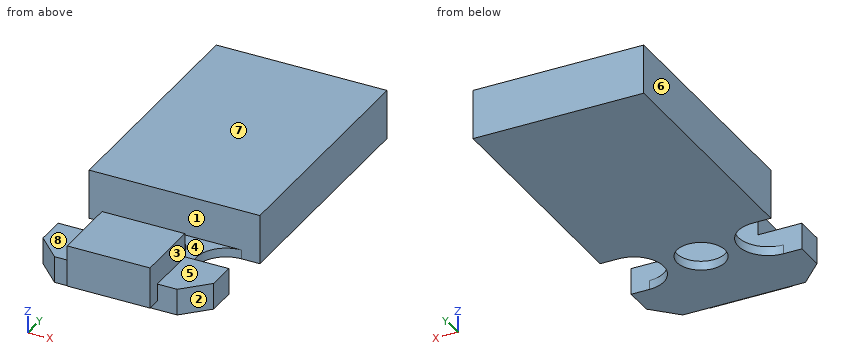
```python
from build123d import *

# Parameters (mm, degrees)
SKETCH1_W           = 20.6
SKETCH1_H           = 43.1
BOSS_EXTRUDE1_DEPTH = 1.1
SKETCH2_W           = 20.6
SKETCH2_H           = 29.5
BOSS_EXTRUDE2_DEPTH = 4.9
SKETCH3_R           = 2.9
CUT_EXTRUDE1_DEPTH  = 4.9
SKETCH4_W           = 10
SKETCH4_H           = 8.1
BOSS_EXTRUDE3_DEPTH = 5
SKETCH5_W           = 20.6
SKETCH5_H           = 6.4
BOSS_EXTRUDE4_DEPTH = 2.1
CUT_EXTRUDE2_DEPTH  = 48.877029983


with BuildPart() as part:
    # Sketch1 → Boss-Extrude1 (new body)
    with BuildSketch(Plane.XY):
        with Locations((10.3, 21.55)):
            Rectangle(SKETCH1_W, SKETCH1_H)
    extrude(amount=BOSS_EXTRUDE1_DEPTH)

    # Sketch2 → Boss-Extrude2 (add)
    with BuildSketch(Plane.XY.offset(1.1)):
        with Locations((10.3, 28.35)):
            Rectangle(SKETCH2_W, SKETCH2_H)
    extrude(amount=BOSS_EXTRUDE2_DEPTH)

    # Sketch3 → Cut-Extrude1 (cut)
    with BuildSketch(Plane.XY.offset(1.1)):
        with Locations((10.3, 10)):
            Circle(SKETCH3_R)
        with BuildLine():
            Line((0, 13.6), (2.2, 13.6))
            ThreePointArc((2.2, 13.6), (5.8, 10), (2.2, 6.4))
            Line((2.2, 6.4), (0, 6.4))
            Line((0, 6.4), (0, 13.6))
        make_face()
        with BuildLine():
            Line((20.6, 13.6), (18.4, 13.6))
            ThreePointArc((18.4, 13.6), (14.8, 10), (18.4, 6.4))
            Line((18.4, 6.4), (20.6, 6.4))
            Line((20.6, 6.4), (20.6, 13.6))
        make_face()
    extrude(amount=-CUT_EXTRUDE1_DEPTH, mode=Mode.SUBTRACT)

    # Sketch4 → Boss-Extrude3 (add)
    with BuildSketch(Plane.XY.offset(1.1)):
        with Locations((10.3, 2.35)):
            Rectangle(SKETCH4_W, SKETCH4_H)
    extrude(amount=BOSS_EXTRUDE3_DEPTH)

    # Sketch5 → Boss-Extrude4 (add)
    with BuildSketch(Plane.XY.offset(1.1)):
        with Locations((10.3, 3.2)):
            Rectangle(SKETCH5_W, SKETCH5_H)
    extrude(amount=BOSS_EXTRUDE4_DEPTH)

    # Sketch6 → Cut-Extrude2 (cut, through all)
    with BuildSketch(Plane.XY.offset(3.2)):
        Polygon((0, 0), (0, 2.9), (2.9, 0), align=None)
        Polygon((20.6, 0), (20.6, 2.9), (17.7, 0), align=None)
    extrude(amount=-CUT_EXTRUDE2_DEPTH, mode=Mode.SUBTRACT)


solid = part.part
```
Geometry check sheet. Reference: the model listing, model coordinates, mm. Face numbers are marked on the shaded views. A direction names the side the tool comes from. Give positions to 0.01 mm unless a question says otherwise; leave off trailing zeros. Write each loop counter-clockwise with the first axis right and the second up, starting at its lowest first coordinate (ties: lowest second). Pieces come first, ordered by that corner, then holes.
1) Material ranges on L1, parallel to Y at x = 10.3, z = 0.35; L2, parallel to Y at x = 14.5, z = 2.25; L3, parallel to Z at x = 8.75, y = 41.5, recorded low to high.
2) Gauge pin test, flat ends, axial feed: pin 1 (1.5 mm diameter, centred on y = 3.5, z = 4, fed in from -X); pin 2 (8 mm diameter, centred on x = 10, y = 37, fed in from +Z); pin 3 (6 mm diameter, centred on x = 2, y = 3, fed in from +Z); pin 4 (9.5 mm diameter, centred on x = 10.3, y = 10, fed in from +Z). Record the tip position at first contact, or that the pin passes through.
3) Section check D-D, the plane y = 5.5. Record the boundary of the cut face in (x, z), and give its area (3 significant figures).
4) Section check B-B, the plane y = 10. Record the boundary of the cut face in (x, z), and give its area (3 significant figures).
5) Access from +Z, -Z, +X, -X, +Y, -Y to the whole of each face (thin tool, end or side, straight path). Record for the marked faces 4, 5, 6, 7 and 8.
6) Release check for a two-part mould opening along Y. For the marked faces 1, 2 and 3 record: pulls with the +Y half, pulls with the -Y half, needs draft (parallel to the pull), parting line crosses it, or undercut.
7) Section check C-C, the plane z = 2.5. Record the boundary of the cut face in (x, y).
8) Section check A-A, the plane x = 10.3. Record the boundary of the cut face in (y, z), and give its area (3 significant figures).
Computed:
1. L1: y = 0 to 7.1, 12.9 to 43.1
1. L2: y = -1.7 to 6.4, 13.6 to 43.1
1. L3: z = 0 to 6
2. pin 1: stops at x = 5.3
2. pin 2: stops at z = 6
2. pin 3: stops at z = 3.2
2. pin 4: stops at z = 6.1
3. outline: (0, 0) - (20.6, 0) - (20.6, 3.2) - (15.3, 3.2) - (15.3, 6.1) - (5.3, 6.1) - (5.3, 3.2) - (0, 3.2) - close
3. area: 94.9 mm2
4. outline: (5.8, 0) - (7.4, 0) - (7.4, 1.1) - (5.8, 1.1) - close; (13.2, 0) - (14.8, 0) - (14.8, 1.1) - (13.2, 1.1) - close
4. area: 3.52 mm2
5. face 4: +Z, +X, -X
5. face 5: +Z, +X, -Y
5. face 6: +Z, -Z, -X, +Y, -Y
5. face 7: +Z, +X, -X, +Y
5. face 8: +Z, -X, -Y
6. face 1: undercut
6. face 2: pulls with the -Y half
6. face 3: needs draft
7. outline: (0, 2.9) - (2.9, 0) - (5.3, 0) - (5.3, -1.7) - (15.3, -1.7) - (15.3, 0) - (17.7, 0) - (20.6, 2.9) - (20.6, 6.4) - (0, 6.4) - close; (0, 13.6) - (20.6, 13.6) - (20.6, 43.1) - (0, 43.1) - close
8. outline: (-1.7, 1.1) - (0, 1.1) - (0, 0) - (7.1, 0) - (7.1, 1.1) - (6.4, 1.1) - (6.4, 6.1) - (-1.7, 6.1) - close; (12.9, 0) - (43.1, 0) - (43.1, 6) - (13.6, 6) - (13.6, 1.1) - (12.9, 1.1) - close
8. area: 226 mm2
